Design review of the part built by this model. Coordinates are the model's own, in mm. Face numbers are marked on the shaded views. A direction names the side the tool comes from. Coordinates: 2 decimals unless noted, no trailing zeros. Loops run counter-clockwise (first coordinate to the right, second up) from the corner with the lowest first, then second, coordinate; pieces in that order, holes last. Notation, with made-up numbers: (3.25, -33.5) - (62.25, -33.5) arc R16 ccw to (62.25, -29.5) - close; hole circle Ø1 at (0, 6). An arc over 180 degrees is marked (long way). One line per question, with ' | ' between items.
Autodesk Inventor part; units mm, degrees
ref_plane "YZ Plane" through (0, 0, 0) normal (1, 0, 0) x (0, 1, 0)
ref_plane "XZ Plane" through (0, 0, 0) normal (0, 1, 0) x (-1, 0, 0)
ref_plane "XY Plane" through (0, 0, 0) normal (0, 0, 1) x (1, 0, 0)
sketch "Sketch1" plane through (0, 0, 0) normal (0, 0, 1) x (1, 0, 0)
  line L0 (-29.3592, 0) -> (29.3592, 0) construction
  line L1 (0, 14.1975) -> (0, -14.1975) construction
  line L2 (-12, 0) -> (12, 0)
  line L3 (12, 0) -> (12, 20)
  line L4 (-12, 20) -> (-12, 0)
  line L5 (-12, 20) -> (-12, 20.8787) construction
  line L6 (12, 20) -> (-12, 20)
  line L7 (50.3592, 10.5) -> (29.3592, 10.5)
  line L8 (29.3592, 10.5) -> (29.3592, -10.5)
  line L9 (29.3592, -10.5) -> (50.3592, -10.5)
  line L10 (50.3592, -10.5) -> (50.3592, 10.5)
  line L11 (29.3592, 0) -> (50.3592, 0) construction
  line L12 (39.8592, 0) -> (39.8592, 3.5595) construction
  circle A0 centre (39.8592, 0) radius 20
  line L13 (33.8592, 10.5) -> (45.8592, 10.5) construction
  line L14 (45.8592, 10.5) -> (45.8592, 24.7953) construction
  line L15 (45.8592, 24.7953) -> (33.8592, 24.7953) construction
  line L16 (33.8592, 24.7953) -> (33.8592, 10.5) construction
  line L17 (33.8592, 18.5) -> (45.8592, 18.5) construction
  point P0 (0, 0)
  point P1 (0, 0)
  point P2 (39.8592, 10.5)
  dimension "d1" = 24
  dimension "d2" = 12
  dimension "d5" = 40
  dimension "d18" = 21
  dimension "d19" = 21
  dimension "d20" = 12
  dimension "d22" = 8
  dimension "d23" = 40
revolve "Revolution1" add sketch "Sketch1" angle 360 about axis through (-29.3592, 0, 0) along (1, 0, 0) contours L4 L6 L3 L2
sketch "Sketch3" plane through (-12, 0, 0) normal (-1, 0, 0) x (0, 0, 1)
  line L0 (-10.5, 10.5) -> (10.5, 10.5)
  line L1 (10.5, 10.5) -> (10.5, -10.5)
  line L2 (10.5, -10.5) -> (-10.5, -10.5)
  line L3 (-10.5, -10.5) -> (-10.5, 10.5)
  point P0 (0, 0)
  point P1 (0, 10.5)
  point P2 (-10.5, 0)
  dimension "d24" = 21
  dimension "d25" = 21
extrude "Extrusion1" cut sketch "Sketch3" against normal through all
fillet "Fillet1" radius 3 4 edges at (0, 10.5, -10.5) (0, -10.5, -10.5) (0, -10.5, 10.5) (0, 10.5, 10.5)
sketch "Sketch4" plane through (-12, 10.5, -7.5) normal (0, -1, 0) x (1, 0, 0)
  point P0 (12, 7.5)
  point P1 (12, 7.5)
hole "Hole2" at (0, 10.5, 0) direction (0, 1, 0) diameter 12 depth 10 tip angle 118
pattern_circular "Circular Pattern2" count 2 over 360 about axis through (0, 0, 0) along (1, 0, 0) of "Hole2"
sketch "Sketch5" plane through (-12, 0, 0) normal (-1, 0, 0) x (0, 0, 1)
  circle A0 centre (0, 0) radius 14
  dimension "d39" = 28
extrude "Extrusion2" cut sketch "Sketch5" against normal blind 1.6
sketch "Sketch6" plane through (12, 0, 0) normal (1, 0, 0) x (0, 0, -1)
  circle A0 centre (0, 0) radius 14
extrude "Extrusion3" cut sketch "Sketch6" against normal blind 1.6
sketch "Sketch7" plane through (12, 0, 0) normal (1, 0, 0) x (0, 0, -1)
  line L0 (-29.6226, 0) -> (29.6226, 0) construction
  line L1 (0, 0) -> (-16.5524, 16.5524) construction
  circle A0 centre (0, 0) radius 17 construction
  point P0 (-12.0208, 12.0208)
  dimension "d45" = 34
  dimension "d44" = 45
hole "Hole3" at (12, 12.0208, 12.0208) direction (-1, 0, 0) diameter 1.567 depth 8 tip angle 118
pattern_circular "Circular Pattern3" count 4 over 360 about axis through (0, 0, 0) along (1, 0, 0) of "Hole3"
mirror "Mirror1" about plane through (0, 0, 0) normal (1, 0, 0) of "Hole3", "Circular Pattern3"
properties part number "P03" material "PVC-U (Transp. / Durchsicht.)"
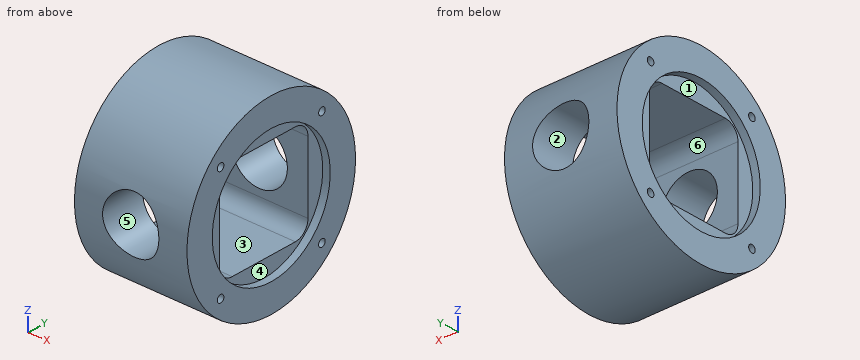
Q1. Tool access review of the marked faces 1, 2 and 3: name each direction out of +Z, -Z, +X, -X, +Y, -Y from which nothing blocks a thin tool from reaching the whole face with its end or side.
Returned:
face 1: -X | face 2: +Y, -Y | face 3: +X, -X
Q2. Take a section at B-B (x = -4.5). Give the boundary of the cut face in (y, z), plus the area to 3 significant figures.
Returned:
outline: (-19.6, -3.97) arc R20 ccw to (19.6, -3.97) - (10.5, -3.97) - (10.5, -7.5) arc R3 cw to (7.5, -10.5) - (-7.5, -10.5) arc R3 cw to (-10.5, -7.5) - (-10.5, -3.97) - close; (-19.6, 3.97) - (-10.5, 3.97) - (-10.5, 7.5) arc R3 cw to (-7.5, 10.5) - (7.5, 10.5) arc R3 cw to (10.5, 7.5) - (10.5, 3.97) - (19.6, 3.97) arc R20 ccw to start; hole circle Ø1.57 at (-12.02, -12.02); hole circle Ø1.57 at (-12.02, 12.02); hole circle Ø1.57 at (12.02, -12.02); hole circle Ø1.57 at (12.02, 12.02) | area: 667 mm²
Q3. Draft analysis for pull direction X (two halves, no side actions). For the marked faces 4, 5 and 6, state which applies: +X half, -X half, draft (parallel to the pull), parting line (faces both ways), or undercut.
Returned:
face 4: +X half | face 5: undercut | face 6: draft
Q4. Take a section at D-D (x = 0). Give the boundary of the cut face in (y, z).
Returned:
outline: (-19.08, -6) arc R20 ccw to (19.08, -6) - (10.5, -6) - (10.5, -7.5) arc R3 cw to (7.5, -10.5) - (-7.5, -10.5) arc R3 cw to (-10.5, -7.5) - (-10.5, -6) - close; (-19.08, 6) - (-10.5, 6) - (-10.5, 7.5) arc R3 cw to (-7.5, 10.5) - (7.5, 10.5) arc R3 cw to (10.5, 7.5) - (10.5, 6) - (19.08, 6) arc R20 ccw to start
Q5. Take a section at C-C (y = 0). Give the boundary of the cut face in (x, z), plus the area to 3 significant figures.
Returned:
outline: (-12, -20) - (12, -20) - (12, -14) - (10.4, -14) - (10.4, -10.5) - (-10.4, -10.5) - (-10.4, -14) - (-12, -14) - close; (-12, 14) - (-10.4, 14) - (-10.4, 10.5) - (10.4, 10.5) - (10.4, 14) - (12, 14) - (12, 20) - (-12, 20) - close | area: 434 mm²
Q6. Take a section at A-A (z = 0). Give the boundary of the cut face in (x, y).
Returned:
outline: (-12, -20) - (-6, -20) - (-6, -10.5) - (-10.4, -10.5) - (-10.4, -14) - (-12, -14) - close; (-12, 14) - (-10.4, 14) - (-10.4, 10.5) - (-6, 10.5) - (-6, 20) - (-12, 20) - close; (6, -20) - (12, -20) - (12, -14) - (10.4, -14) - (10.4, -10.5) - (6, -10.5) - close; (6, 10.5) - (10.4, 10.5) - (10.4, 14) - (12, 14) - (12, 20) - (6, 20) - close
Q7. For pin 1 (2.5 mm diameter, centred on y = -12.02, z = -12.02, fed in from -X); pin 2 (8 mm diameter, centred on x = 3, y = -8.5, fed in from -Z); pin 3 (3 mm diameter, centred on x = 2, z = -7, fed in from +Y); pin 4 (7.5 mm diameter, centred on x = 1.5, z = 2, fed in from -Y), all flat-tipped, find the tip position at first contact; note any pin that passes through.
Returned:
pin 1: stops at x = -12 | pin 2: stops at z = -19.49 | pin 3: stops at y = 19.22 | pin 4: stops at y = -19.73
Q8. To check wall thickness, follow line 1 along X through (y, z) = (17, 0); line 2 along X through (y, z) = (7, 11.5); line 3 along Y through (x, z) = (-2.75, -6). State the ranges of each line that lie inside material, in increasing order.
Returned:
line 1: x = -12 to -6, 6 to 12 | line 2: x = -10.4 to 10.4 | line 3: y = -19.08 to -10.5, 10.5 to 19.08
